```python
from build123d import *

# Parameters (mm, degrees)
SKETCH1_R               = 6.5
BOSS_EXTRUDE1_DEPTH     = 20
BOSS_EXTRUDE2_DEPTH     = 42
SKETCH4_W               = 40
SKETCH4_H               = 20
CUT_EXTRUDE1_DEPTH      = 25
BOSS_EXTRUDE3_DEPTH     = 11
FILLET1_R               = 3
SKETCH7_R               = 15
SKETCH7_R_2             = 10
BOSS_EXTRUDE4_DEPTH     = 18
FILLET2_R               = 1
CUT_EXTRUDE2_START      = -94
SKETCH8_R               = 10
CUT_EXTRUDE2_DEPTH      = 94
CUT_EXTRUDE3_DEPTH      = 199.421269084
CUT_EXTRUDE3_DEPTH_BACK = 199.421269084
SKETCH9_R               = 4


with BuildPart() as part:
    # Sketch1 → Boss-Extrude1 (new body)
    with BuildSketch(Plane(origin=(0, 0, 0), x_dir=(1, 0, 0), z_dir=(0, 1, 0))):
        with BuildLine():
            Line((80, -30), (-80, -30))
            ThreePointArc((-80, -30), (-83.535533906, -28.535533906), (-85, -25))
            Line((-85, -25), (-85, 25))
            ThreePointArc((-85, 25), (-83.535533906, 28.535533906), (-80, 30))
            Line((-80, 30), (80, 30))
            ThreePointArc((80, 30), (83.535533906, 28.535533906), (85, 25))
            Line((85, 25), (85, -25))
            ThreePointArc((85, -25), (83.535533906, -28.535533906), (80, -30))
        make_face()
        with Locations(Location((-70, 0, 0), (0, 0, 270))):
            Circle(SKETCH1_R, mode=Mode.SUBTRACT)
        with Locations(Location((70, 0, 0), (0, 0, 90))):
            Circle(SKETCH1_R, mode=Mode.SUBTRACT)
    extrude(amount=BOSS_EXTRUDE1_DEPTH)

    # Sketch2 → Boss-Extrude2 (add)
    with BuildSketch(Plane.XY.offset(12)):
        with BuildLine():
            Line((15, 20.991212976), (-7, 45))
            Line((-7, 45), (-7, 85))
            Line((-7, 85), (45, 85))
            Line((45, 85), (45, 157))
            Line((45, 157), (-15, 157))
            Line((-15, 157), (-15, 117.662812973))
            ThreePointArc((-15, 117.662812973), (-40.565276927, 93.726843908), (-50, 60))
            Line((-50, 60), (-50, 20))
            Line((-50, 20), (-40, 20))
            Line((-40, 20), (-40, 60))
            ThreePointArc((-40, 60), (-35.707494515, 81.301408404), (-23.5, 99.277856357))
            ThreePointArc((-23.5, 99.277856357), (-18.063508327, 100.316914371), (-15, 95.707142143))
            Line((-15, 95.707142143), (-15, 20))
            Line((-15, 20), (45, 20))
            Line((45, 20), (45, 45))
            Line((45, 45), (37, 45))
            Line((37, 45), (15, 20.991212976))
        make_face()
    extrude(amount=-BOSS_EXTRUDE2_DEPTH)

    # Sketch4 → Cut-Extrude1 (cut)
    with BuildSketch(Plane(origin=(0, 45, 0), x_dir=(1, 0, 0), z_dir=(0, 1, 0))):
        with Locations((15, 9)):
            Rectangle(SKETCH4_W, SKETCH4_H)
    extrude(amount=-CUT_EXTRUDE1_DEPTH, mode=Mode.SUBTRACT)

    # Sketch5 → Boss-Extrude3 (add, symmetric)
    with BuildSketch(Plane.XY.offset(-9)):
        with BuildLine():
            Line((-15, 20), (-15, 95.707142143))
            ThreePointArc((-15, 95.707142143), (-18.063508327, 100.316914371), (-23.5, 99.277856357))
            ThreePointArc((-23.5, 99.277856357), (-35.707494515, 81.301408404), (-40, 60))
            Line((-40, 60), (-40, 20))
            Line((-40, 20), (-15, 20))
        make_face()
    extrude(amount=BOSS_EXTRUDE3_DEPTH, both=True)

    # Fillet1
    fillet1_edges = [part.edges().sort_by_distance(p)[0] for p in [
        (-7, 85, -9),
        (45, 85, -9),
        (45, 157, -9),
        (-15, 157, -9),
    ]]
    fillet(fillet1_edges, radius=FILLET1_R)

    # Sketch7 → Boss-Extrude4 (add)
    with BuildSketch(Plane(origin=(0, 157, 0), x_dir=(1, 0, 0), z_dir=(0, 1, 0))):
        with Locations(Location((15, 9, 0), (0, 0, 270))):
            Circle(SKETCH7_R)
        with Locations(Location((15, 9, 0), (0, 0, 270))):
            Circle(SKETCH7_R_2, mode=Mode.SUBTRACT)
    extrude(amount=BOSS_EXTRUDE4_DEPTH)

    # Fillet2
    fillet2_edges = [part.edges().sort_by_distance(p)[0] for p in [
        (15, 157, -24),
        (45, 20, -9),
        (15, 20, 12),
        (-50, 20, -9),
        (-45, 20, 12),
        (-40, 20, 7),
        (-15, 20, 7),
    ]]
    fillet(fillet2_edges, radius=FILLET2_R)

    # Sketch8 → Cut-Extrude2 (cut)
    with BuildSketch(Plane(origin=(0, 157, 0), x_dir=(1, 0, 0), z_dir=(0, 1, 0)).offset(CUT_EXTRUDE2_START)):
        with Locations(Location((15, 9, 0), (0, 0, 90))):
            Circle(SKETCH8_R)
    extrude(amount=CUT_EXTRUDE2_DEPTH, mode=Mode.SUBTRACT)

    # Sketch9 → Cut-Extrude3 (cut, two sides: drawn at the far end of the back side and taken through both)
    with BuildSketch(Plane(origin=(0, 0, -9), x_dir=(0, 0, -1), z_dir=(1, 0, 0)).offset(-CUT_EXTRUDE3_DEPTH_BACK)):
        with Locations(Location((0, 140, 0), (0, 0, 180))):
            Circle(SKETCH9_R)
    extrude(amount=CUT_EXTRUDE3_DEPTH + CUT_EXTRUDE3_DEPTH_BACK, mode=Mode.SUBTRACT)


solid = part.part
```
Geometry: final body of the model. Coordinates: model frame, mm. A direction names the side the tool comes from. Coordinates: 2 decimals unless noted, no trailing zeros. Order: outer loops, then holes, each group sorted by start corner. A loop starts at its lowest first (then second) coordinate and runs counter-clockwise, first axis right, second up. Notation, with made-up numbers: (-3, -27) - (3, -27) arc R8 cw to (3, -16) - close; hole circle Ø6 at (-10, 71). An arc over 180 degrees is marked (long way). Return JSON: item names as keys, results as strings. Group by question number.
1. Cut plane A-A (y = 140). Output: boundary loops of the cut face in (x, z).
2. Cut plane D-D (y = 49). Output: boundary loops of the cut face in (x, z), plus the area to 3 significant figures.
3. Pin query (flat end, axial travel): pin 1 (8 mm diameter, centred on y = 67, z = 5.5, fed in from -X); pin 2 (10 mm diameter, centred on y = 102.5, z = -12.5, fed in from +X); pin 3 (5 mm diameter, centred on y = 52.5, z = -24.5, fed in from -X). Return the tip coordinate at first contact, or that it passes through.
4. Cut plane C-C (z = -9). Count the separate pieces of the cut face and the enclosed holes in it, plus the area to 3 significant figures.
5. Set-up query: faces 1 (the face through (-5, 32, -9)), 2 (the face through (-15, 132, -9)), 3 (the face through (-5.624, 43.498, -8.706)). Return all of +Z, -Z, +X, -X, +Y, -Y with unobstructed straight access to the full face (end or side cutting, diameter ignored); none if empty.
6. Cut plane B-B (x = 70). Output: boundary loops of the cut face in (y, z).
7. Pull-direction query (X, two-part tool) for faces 4 (the face through (1, 10, 30)), 5 (the face through (35, 32, -9)), 6 (the face through (45, 33, -9)); classes: pulls with the +X half, pulls with the -X half, needs draft (parallel to the pull), parting line crosses it, or undercut.
8. Material intervals for line 1 along X through (y, z) = (7.5, 0); line 2 along X through (y, z) = (150, -8.5); line 3 along Z through (x, y) = (-5.5, 140), sorted ascending. Write a range as [from, to].
Resolved:
{
 "1": {"outline": "(-15, -30) - (45, -30) - (45, -13) - (24.17, -13) arc R10 cw to (5.83, -13) - (-15, -13) - close; (-15, -5) - (5.83, -5) arc R10 cw to (24.17, -5) - (45, -5) - (45, 12) - (-15, 12) - close"},
 "2": {"outline": "(-50, -30) - (-40, -30) - (-40, -20) - (-15, -20) - (-15, -30) - (-7, -30) - (-7, 12) - (-15, 12) - (-15, 2) - (-40, 2) - (-40, 12) - (-50, 12) - close", "area": "1,310 mm²"},
 "3": {"pin 1": "stops at x = -49.93", "pin 2": "stops at x = 45", "pin 3": "stops at x = -50"},
 "4": {"separate pieces": "4", "enclosed holes": "0", "area": "9,790 mm²"},
 "5": {"face 1": "none", "face 2": "+Z, -Z, -X, +Y", "face 3": "+Z, -Z"},
 "6": {"outline": "(0, -30) - (20, -30) - (20, -6.5) - (0, -6.5) - close; (0, 6.5) - (20, 6.5) - (20, 30) - (0, 30) - close"},
 "7": {"face 4": "needs draft", "face 5": "undercut", "face 6": "pulls with the +X half"},
 "8": {"line 1": "x = [-85, -76.5], [-63.5, 63.5], [76.5, 85]", "line 2": "x = [-15, 5.01], [24.99, 45]", "line 3": "z = [-30, -13], [-5, 12]"}
}
